The listing builds one solid part. Answer for the finished solid, in the listing's coordinates (mm). Face numbers are marked on the shaded views. Give positions to 0.01 mm unless a question says otherwise; leave off trailing zeros. Write each loop counter-clockwise with the first axis right and the second up, starting at its lowest first coordinate (ties: lowest second). Pieces come first, ordered by that corner, then holes. Notation, with made-up numbers: (69, -12) - (116, -12) arc R19 ccw to (116, 8) - close; hole circle Ø7 at (8, 53.5). An arc over 180 degrees is marked (long way). One line per question, with ' | ' between items. Start each with the question number.
1. Find the intervals of material crossed by L1, parallel to Y at x = 0, z = -4; L2, parallel to X at y = 16, z = -5.25; L3, parallel to Z at x = 32, y = 12.5, in increasing order. Write a range as from..to.
2. A cutting plane is placed at C-C (z = -3.25). Determine the outline of the cut face in (x, y).
3. A cutting plane is placed at A-A (x = 0). Determine the outline of the cut face in (y, z), then the cut area to 4 significant figures.
4. The mould has two halves that part along X. Classify the marked faces 1, 2 and 3: +X half, -X half, draft (parallel to the pull), parting line (faces both ways), or undercut.
5. A cutting plane is placed at B-B (y = 0). Determine the outline of the cut face in (x, z), then the cut area to 3 significant figures.
6. A cutting plane is placed at D-D (y = -31.5). Determine the outline of the cut face in (x, z).
7. Given P1, Ø5.5, axis at x = 0, y = -32, coming from the -Z side; P2, Ø3, axis at y = 30, z = -4, coming from the +X side (3 decimals); P3, Ø1, axis at y = 3.5, z = -6, coming from the -X side, each flat-ended and moving along its own axis, determine where each tip first touches the part or whether it passes through.
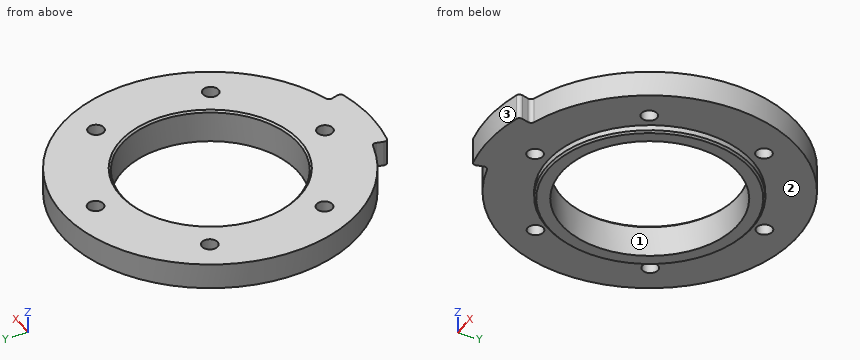
Autodesk Inventor part; units mm, degrees
ref_plane "YZ Plane" through (0, 0, 0) normal (1, 0, 0) x (0, 1, 0)
ref_plane "XZ Plane" through (0, 0, 0) normal (0, 1, 0) x (-1, 0, 0)
ref_plane "XY Plane" through (0, 0, 0) normal (0, 0, 1) x (1, 0, 0)
sketch "スケッチ2" plane through (0, 0, 0) normal (1, 0, 0) x (0, 1, 0)
  line L0 (24.1, 0) -> (24.1, -9)
  line L1 (40.5, 0) -> (40.5, -7)
  line L2 (40.5, 0) -> (24.1, 0)
  line L3 (24.1, 0) -> (59, 0)
  line L4 (24.1, -9) -> (28, -9)
  line L5 (0, -10.8) -> (0, 1.8)
  line L6 (28, -9) -> (28, -7)
  line L7 (28, -7) -> (40.5, -7)
  point P0 (0, 0)
  dimension "d40" = 24.1
  dimension "d41" = 7
  dimension "d42" = 40.5
  dimension "d43" = 28
  dimension "d44" = 2
revolve "回転1" add sketch "スケッチ2" angle 360 about axis through (0, 0, -10) along (0, 0, 1)
sketch "スケッチ4" plane through (0, 0, 0) normal (0, 0, 1) x (1, 0, 0)
  point P0 (0, 0)
  point P1 (0, 32)
  point P2 (-27.7128, 16)
  point P3 (-27.7128, -16)
  point P4 (0, -32)
  point P5 (27.7128, -16)
  point P6 (27.7128, 16)
  dimension "d11" = 32
  dimension "d14" = 360
hole "穴1" at (0, 32, 0) at (-27.7128, 16, 0) at (-27.7128, -16, 0) at (0, -32, 0) at (27.7128, -16, 0) at (27.7128, 16, 0) direction (0, 0, -1) diameter 4.3 end through all
chamfer "面取り3" distance 0.5 angle 45 1 edges at (0, -28, -9)
chamfer "面取り4" distance 0.5 angle 45 1 edges at (0, -24.1, 0)
sketch "スケッチ7" plane through (0, 0, 0) normal (0, 0, 1) x (1, 0, 0)
  circle A0 centre (0, 0) radius 40.5
  circle A1 centre (0, 0) radius 44.5
  line L0 (0, 0) -> (11.5174, -42.9837)
  line L1 (0, 0) -> (-11.5174, -42.9837)
  line L2 (0, 62.3) -> (0, -62.3)
  point P0 (10.4822, -39.12)
  point P1 (-10.4822, -39.12)
  dimension "d51" = 4
  dimension "d52" = 15
  dimension "d53" = 15
extrude "押し出し3" add sketch "スケッチ7" against normal up to surface (7 mm away) contours L0 A1 L2 A0 | A0 L2 A1 L1 picked at (6.2128, -42.6798) picked at (-1.2928, -43.1102)
fillet "フィレット1" radius 1 4 edges at (10.4822, -39.12, -3.5) (11.5174, -42.9837, -3.5) (-10.4822, -39.12, -3.5) (-11.5174, -42.9837, -3.5)
properties part number "base12" material "ABS プラスチック"
Determined:
1) L1: -44.5..-34.15, -29.85..-24.1, 24.1..29.85, 34.15..40.5 | L2: -37.21..-29.86, -25.56..-18.02, 18.02..25.56, 29.86..37.21 | L3: -7..0
2) outline: (-11.42, -38.86) arc R1 cw to (-10.74, -40.07) - (-11.26, -42.01) arc R1 ccw to (-10.53, -43.24) arc R44.5 ccw to (10.53, -43.24) arc R1 ccw to (11.26, -42.01) - (10.74, -40.07) arc R1 cw to (11.42, -38.86) arc R40.5 ccw (long way) to start; hole circle Ø4.3 at (-27.71, -16); hole circle Ø4.3 at (-27.71, 16); hole circle Ø48.2 at (0, 0); hole circle Ø4.3 at (0, -32); hole circle Ø4.3 at (0, 32); hole circle Ø4.3 at (27.71, -16); hole circle Ø4.3 at (27.71, 16)
3) outline: (-44.5, -7) - (-34.15, -7) - (-34.15, 0) - (-44.5, 0) - close; (-29.85, -7) - (-28, -7) - (-28, -8.5) - (-27.5, -9) - (-24.1, -9) - (-24.1, -0.5) - (-24.6, 0) - (-29.85, 0) - close; (24.1, -9) - (27.5, -9) - (28, -8.5) - (28, -7) - (29.85, -7) - (29.85, 0) - (24.6, 0) - (24.1, -0.5) - close; (34.15, -7) - (40.5, -7) - (40.5, 0) - (34.15, 0) - close | area: 212.5 mm2
4) face 1: undercut | face 2: draft | face 3: parting line
5) outline: (-40.5, -7) - (-28, -7) - (-28, -8.5) - (-27.5, -9) - (-24.1, -9) - (-24.1, -0.5) - (-24.6, 0) - (-40.5, 0) - close; (24.1, -9) - (27.5, -9) - (28, -8.5) - (28, -7) - (40.5, -7) - (40.5, 0) - (24.6, 0) - (24.1, -0.5) - close | area: 245 mm2
6) outline: (-25.46, -7) - (-2.09, -7) - (-2.09, 0) - (-25.46, 0) - close; (2.09, -7) - (25.46, -7) - (25.46, 0) - (2.09, 0) - close
7) P1: z = -7 | P2: x = 28.775 | P3: x = -40.39
